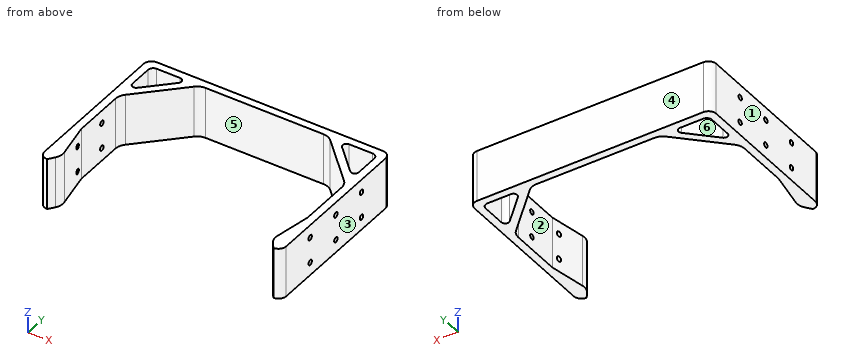
```python
from build123d import *

# Parameters (mm, degrees)
BOSS_EXTRUDE2_DEPTH = 20
SKETCH2_R           = 1
CUT_EXTRUDE1_DEPTH  = 5


with BuildPart() as part:
    # Sketch1 → Boss-Extrude2 (new body)
    with BuildSketch(Plane.XY):
        with BuildLine():
            ThreePointArc((-47, -29), (-46.121320344, -31.121320344), (-44, -32))
            Line((-44, -32), (-42.320425457, -29.72852746))
            ThreePointArc((-42.320425457, -29.72852746), (-41.468325666, -27.878092848), (-41.42508346, -25.841352212))
            Line((-41.42508346, -25.841352212), (-44, -12))
            Line((-44, -12), (-44, 7.928932188))
            ThreePointArc((-44, 7.928932188), (-43.619397663, 9.84234935), (-42.535533906, 11.464466094))
            Line((-42.535533906, 11.464466094), (-26.464466094, 27.535533906))
            ThreePointArc((-26.464466094, 27.535533906), (-24.84234935, 28.619397663), (-22.928932188, 29))
            Line((-22.928932188, 29), (22.928932188, 29))
            ThreePointArc((22.928932188, 29), (24.84234935, 28.619397663), (26.464466094, 27.535533906))
            Line((26.464466094, 27.535533906), (42.535533906, 11.464466094))
            ThreePointArc((42.535533906, 11.464466094), (43.619397663, 9.84234935), (44, 7.928932188))
            Line((44, 7.928932188), (44, -12))
            Line((44, -12), (41.42508346, -25.841352212))
            ThreePointArc((41.42508346, -25.841352212), (41.468325666, -27.878092848), (42.320425457, -29.72852746))
            Line((42.320425457, -29.72852746), (44, -32))
            ThreePointArc((44, -32), (46.121320344, -31.121320344), (47, -29))
            Line((47, -29), (47, 29))
            ThreePointArc((47, 29), (46.121320344, 31.121320344), (44, 32))
            Line((44, 32), (-44, 32))
            ThreePointArc((-44, 32), (-46.121320344, 31.121320344), (-47, 29))
            Line((-47, 29), (-47, -29))
        make_face()
        with BuildLine():
            ThreePointArc((-44, 27), (-43.414213562, 28.414213562), (-42, 29))
            Line((-42, 29), (-32.863961031, 29))
            ThreePointArc((-32.863961031, 29), (-31.478141732, 28.074025149), (-31.803300859, 26.439339828))
            Line((-31.803300859, 26.439339828), (-41.439339828, 16.803300859))
            ThreePointArc((-41.439339828, 16.803300859), (-43.074025149, 16.478141732), (-44, 17.863961031))
            Line((-44, 17.863961031), (-44, 27))
        make_face(mode=Mode.SUBTRACT)
        with BuildLine():
            ThreePointArc((42, 29), (43.414213562, 28.414213562), (44, 27))
            Line((44, 27), (44, 17.863961031))
            ThreePointArc((44, 17.863961031), (43.074025149, 16.478141732), (41.439339828, 16.803300859))
            Line((41.439339828, 16.803300859), (31.803300859, 26.439339828))
            ThreePointArc((31.803300859, 26.439339828), (31.478141732, 28.074025149), (32.863961031, 29))
            Line((32.863961031, 29), (42, 29))
        make_face(mode=Mode.SUBTRACT)
    extrude(amount=BOSS_EXTRUDE2_DEPTH)

    # Sketch2 → Cut-Extrude1 (cut)
    with BuildSketch(Plane.ZY.offset(47)):
        with Locations((5, 15)):
            Circle(SKETCH2_R)
        with Locations((15, 15)):
            Circle(SKETCH2_R)
        with Locations((15, 0)):
            Circle(SKETCH2_R)
        with Locations((15, -15)):
            Circle(SKETCH2_R)
        with Locations((5, 0)):
            Circle(SKETCH2_R)
        with Locations((5, -15)):
            Circle(SKETCH2_R)
    cut_extrude1 = extrude(amount=-CUT_EXTRUDE1_DEPTH, mode=Mode.SUBTRACT)

    # Mirror1: Cut-Extrude1 across plane
    add(cut_extrude1.mirror(Plane(origin=(0, 0, 0), x_dir=(0, 0, 1), z_dir=(1, 0, 0))), mode=Mode.SUBTRACT)


solid = part.part
```
Input: part model. Units: mm. Frame: model coordinates. Face numbers are marked on the shaded views. A direction names the side the tool comes from. Give positions to 0.01 mm unless a question says otherwise; leave off trailing zeros. Order: outer loops, then holes, each group sorted by start corner. A loop starts at its lowest first (then second) coordinate and runs counter-clockwise, first axis right, second up. Notation, with made-up numbers: M 66.25,55 L 85.25,55 A22 cw 85.25,74 Z; hole C -22.5,60 d10. An arc over 180 degrees is marked long. One line per question, with ' | ' between items. Start each with the question number.
1. Access query for the marked faces 4, 5 and 6. Directions: +Z, -Z, +X, -X, +Y, -Y. A direction counts if a zero-diameter tool reaches every point of the face in a straight line with its end or side. Return the directions, or none.
2. Section query D-D (y = 22). Return the cut outline in (x, z).
3. Material intervals for probe 1 along Y at (x, z) = (-44.2, 15); probe 2 along Z at (x, y) = (45, 0); probe 3 along X at (y, z) = (4, 4.5), sorted ascending. Write a range as [from, to].
4. Section query C-C (x = 36.5). Return the cut outline in (y, z).
5. Section query B-B (z = 18). Count the separate pieces of the cut face and the enclosed holes in it, and give its area (3 significant figures).
6. Pull-direction query (X, two-part tool) for the marked faces 1, 2 and 3; classes: released by +X, released by -X, zero draft, split by the parting line, or undercut.
7. First-contact query: pin 1 Ø1.5 at (x, z) = (5, 2.5) entering from -Y; pin 2 Ø1.2 at (y, z) = (0, 15) entering from -X; pin 3 Ø2.5 at (y, z) = (15, 15) entering from +X; pin 4 Ø1.6 at (y, z) = (15, 5) entering from +X. Flat tips, straight axial feed; report the tip coordinate or a pass-through.
8. Section query A-A (y = 0). Return the cut outline in (x, z), and give its area (3 significant figures).
Here are the results:
1) face 4: +Z, -Z, +X, -X, +Y | face 5: +Z, -Z, -Y | face 6: +Z, -Z
2) outline: M -47,0 L -44,0 L -44,20 L -47,20 Z; M -36.24,0 L -32,0 L -32,20 L -36.24,20 Z; M 32,0 L 36.24,0 L 36.24,20 L 32,20 Z; M 44,0 L 47,0 L 47,20 L 44,20 Z
3) probe 1: [-31.99, -16], [-14, -1], [1, 14], [16, 31.99] | probe 2: [0, 4], [6, 14], [16, 20] | probe 3: [-47, -44], [44, 47]
4) outline: M 17.5,0 L 21.74,0 L 21.74,20 L 17.5,20 Z; M 29,0 L 32,0 L 32,20 L 29,20 Z
5) separate pieces: 1 | enclosed holes: 2 | area: 857 mm²
6) face 1: released by -X | face 2: undercut | face 3: released by +X
7) pin 1: y = 29 | pin 2: through | pin 3: x = 47 | pin 4: x = 42
8) outline: M -47,0 L -44,0 L -44,4 L -47,4 Z; M -47,6 L -44,6 L -44,14 L -47,14 Z; M -47,16 L -44,16 L -44,20 L -47,20 Z; M 44,0 L 47,0 L 47,4 L 44,4 Z; M 44,6 L 47,6 L 47,14 L 44,14 Z; M 44,16 L 47,16 L 47,20 L 44,20 Z | area: 96.0 mm²
